Source: CAD feature listing. Evaluate the final solid. Frame: model axes, mm. Face numbers are marked on the shaded views. A direction names the side the tool comes from. Coordinates: 2 decimals unless noted, no trailing zeros. Order: outer loops, then holes, each group sorted by start corner. A loop starts at its lowest first (then second) coordinate and runs counter-clockwise, first axis right, second up. Notation, with made-up numbers: (8, 62) -> (34, 62) arc R21 cw to (34, 79) -> close; hole circle Ø1 at (86.5, 8). An arc over 180 degrees is marked (long way). Write each question's results on one line, items separated by ' | '. Start each with the question number.
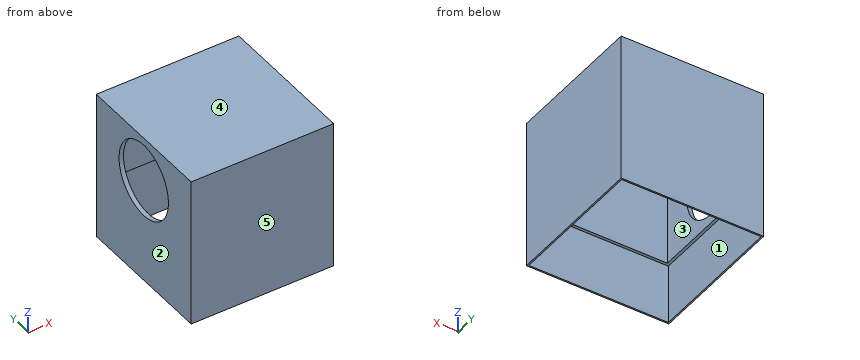
from build123d import *

# Parameters (mm, degrees)
CROQUIS2_W              = 480
CROQUIS2_H              = 505
SALIENTE_EXTRUIR1_DEPTH = 480
CROQUIS3_W              = 470
CROQUIS3_H              = 470
CORTAR_EXTRUIR1_DEPTH   = 200
CROQUIS5_W              = 450
CROQUIS5_H              = 450
CORTAR_EXTRUIR2_DEPTH   = 300
CROQUIS7_R              = 125
CORTAR_EXTRUIR3_DEPTH   = 300


with BuildPart() as part:
    # Croquis2 → Saliente-Extruir1 (new body)
    with BuildSketch(Plane(origin=(0, 0, 0), x_dir=(1, 0, 0), z_dir=(0, 1, 0))):
        Rectangle(CROQUIS2_W, CROQUIS2_H)
    extrude(amount=SALIENTE_EXTRUIR1_DEPTH)

    # Croquis3 → Cortar-Extruir1 (cut)
    with BuildSketch(Plane(origin=(0, 0, -252.5), x_dir=(-1, 0, 0), z_dir=(0, 0, -1))):
        with Locations((0, 240)):
            Rectangle(CROQUIS3_W, CROQUIS3_H)
    extrude(amount=-CORTAR_EXTRUIR1_DEPTH, mode=Mode.SUBTRACT)

    # Croquis5 → Cortar-Extruir2 (cut)
    with BuildSketch(Plane(origin=(0, 0, -52.5), x_dir=(-1, 0, 0), z_dir=(0, 0, -1))):
        with Locations((0, 240)):
            Rectangle(CROQUIS5_W, CROQUIS5_H)
    extrude(amount=-CORTAR_EXTRUIR2_DEPTH, mode=Mode.SUBTRACT)

    # Croquis7 → Cortar-Extruir3 (cut)
    with BuildSketch(Plane.ZY.offset(240)):
        with Locations((102.5, 240)):
            Circle(CROQUIS7_R)
    extrude(amount=-CORTAR_EXTRUIR3_DEPTH, mode=Mode.SUBTRACT)


solid = part.part
(1) Section D-D on y = 391.5. Return the cut outline in (x, z), then the cut area to 3 significant figures.
(2) First-contact query: P1, Ø6, axis at x = 78.5, y = 75, coming from the -Z side; P2, Ø6, axis at x = -25, z = 57, coming from the -Y side. Flat tips, straight axial feed; report the tip coordinate or a pass-through.
(3) Section A-A on y = 240. Return the cut outline in (x, z).
(4) Line query: L1, parallel to X at y = 119, z = -10; L2, parallel to X at y = 289, z = -208; L3, parallel to Y at x = -235, z = 102.5. Output: solid intervals per line, ascending.
(5) Draft query along Y for the marked faces 3, 4 and 5. Return one class per face: released by +Y, released by -Y, zero draft, split by the parting line, or undercut.
(6) Section C-C on x = -118. Return the cut outline in (y, z), then the cut area to 3 significant figures.
(7) Reachability of the marked faces 1 and 2 from +Z, -Z, +X, -X, +Y, -Y: full face, straight path, thin tool, end or side. Return the list, or none.
(8) Section B-B on z = -136.5. Return the cut outline in (x, y), then the cut area to 3 significant figures.
Results list:
1) outline: (-240, -252.5) -> (-235, -252.5) -> (-235, -52.5) -> (-225, -52.5) -> (-225, 247.5) -> (225, 247.5) -> (225, -52.5) -> (235, -52.5) -> (235, -252.5) -> (240, -252.5) -> (240, 252.5) -> (-240, 252.5) -> close | area: 13,400 mm²
2) P1: stops at z = 247.5 | P2: stops at y = 0
3) outline: (-240, -252.5) -> (-235, -252.5) -> (-235, -52.5) -> (-225, -52.5) -> (-225, -22.5) -> (-240, -22.5) -> close; (-240, 227.5) -> (-225, 227.5) -> (-225, 247.5) -> (225, 247.5) -> (225, -52.5) -> (235, -52.5) -> (235, -252.5) -> (240, -252.5) -> (240, 252.5) -> (-240, 252.5) -> close
4) L1: x = -240 to -225, 225 to 240 | L2: x = -240 to -235, 235 to 240 | L3: y = 0 to 115, 365 to 480
5) face 3: undercut | face 4: zero draft | face 5: released by -Y
6) outline: (0, -252.5) -> (5, -252.5) -> (5, -52.5) -> (15, -52.5) -> (15, 247.5) -> (465, 247.5) -> (465, -52.5) -> (475, -52.5) -> (475, -252.5) -> (480, -252.5) -> (480, 252.5) -> (0, 252.5) -> close | area: 13,400 mm²
7) face 1: -Z | face 2: +Z, -Z, -X, +Y, -Y
8) outline: (-240, 0) -> (240, 0) -> (240, 480) -> (-240, 480) -> close; hole (-235, 5) -> (235, 5) -> (235, 475) -> (-235, 475) -> close | area: 9,500 mm²
